```python
from build123d import *

# Parameters (mm, degrees)
F0_W     = 110
F0_H     = 120
F1_DEPTH = 2
F2_R     = 1.5
F3_W     = 2
F3_H     = 2
F3_R     = 1.75
F4_DEPTH = 2
F5_R     = 3


with BuildPart() as f1:
    # F0 (on Top) → F1 (new body)
    with BuildSketch(Plane.XY):
        Rectangle(F0_W, F0_H)
        with BuildLine():
            ThreePointArc((-50, 52.75), (-51.5909902577, 56.5909902577), (-47.75, 55))
            Line((-47.75, 55), (47.75, 55))
            ThreePointArc((47.75, 55), (50, 57.25), (52.25, 55))
            ThreePointArc((52.25, 55), (51.5909902577, 53.4090097423), (50, 52.75))
            Line((50, 52.75), (50, -42.75))
            ThreePointArc((50, -42.75), (51.5909902577, -43.4090097423), (52.25, -45))
            ThreePointArc((52.25, -45), (50, -47.25), (47.75, -45))
            Line((47.75, -45), (-47.75, -45))
            ThreePointArc((-47.75, -45), (-51.5909902577, -46.5909902577), (-50, -42.75))
            Line((-50, -42.75), (-50, 52.75))
        make_face(mode=Mode.SUBTRACT)
        with BuildLine():
            Line((47.75, 55), (-47.75, 55))
            ThreePointArc((-47.75, 55), (-48.4090097423, 53.4090097423), (-50, 52.75))
            Line((-50, 52.75), (-50, -42.75))
            ThreePointArc((-50, -42.75), (-48.4090097423, -43.4090097423), (-47.75, -45))
            Line((-47.75, -45), (47.75, -45))
            ThreePointArc((47.75, -45), (48.4090097423, -43.4090097423), (50, -42.75))
            Line((50, -42.75), (50, 52.75))
            ThreePointArc((50, 52.75), (48.4090097423, 53.4090097423), (47.75, 55))
        make_face()
    extrude(amount=F1_DEPTH)

    # F2
    f2_edges = [f1.edges().sort_by_distance(p)[0] for p in [
        (55, 60, 1),
        (55, -60, 1),
        (-55, -60, 1),
        (-55, 60, 1),
    ]]
    fillet(f2_edges, radius=F2_R)

    # F3 (on face) → F4 (cut)
    with BuildSketch(Plane.XY.offset(2)):
        with Locations((-24, 1)):
            Rectangle(F3_W, F3_H)
        with Locations((-26, 1)):
            Rectangle(F3_W, F3_H)
        with BuildLine():
            Line((-27, 2), (-25, 2))
            Line((-25, 2), (-23, 2))
            Line((-23, 2), (-23, 7.5))
            ThreePointArc((-23, 7.5), (-25, 9.5), (-27, 7.5))
            Line((-27, 7.5), (-27, 2))
        make_face()
        with Locations((-24, -1)):
            Rectangle(F3_W, F3_H)
        with Locations((-26, -1)):
            Rectangle(F3_W, F3_H)
        with BuildLine():
            Line((-27, 0), (-27, 2))
            Line((-27, 2), (-32.5, 2))
            ThreePointArc((-32.5, 2), (-34.5, 0), (-32.5, -2))
            Line((-32.5, -2), (-27, -2))
            Line((-27, -2), (-27, 0))
        make_face()
        with BuildLine():
            Line((-17.5, 2), (-23, 2))
            Line((-23, 2), (-23, 0))
            Line((-23, 0), (-23, -2))
            Line((-23, -2), (-17.5, -2))
            ThreePointArc((-17.5, -2), (-15.5, 0), (-17.5, 2))
        make_face()
        with BuildLine():
            Line((-23, -2), (-25, -2))
            Line((-25, -2), (-27, -2))
            Line((-27, -2), (-27, -7.5))
            ThreePointArc((-27, -7.5), (-25, -9.5), (-23, -7.5))
            Line((-23, -7.5), (-23, -2))
        make_face()
        Circle(F3_R)
        with BuildLine():
            Line((23, 2), (17.5, 2))
            ThreePointArc((17.5, 2), (15.5, 0), (17.5, -2))
            Line((17.5, -2), (23, -2))
            Line((23, -2), (23, 0))
            Line((23, 0), (23, 2))
        make_face()
        with BuildLine():
            Line((23, 7.5), (23, 2))
            Line((23, 2), (25, 2))
            Line((25, 2), (27, 2))
            Line((27, 2), (27, 7.5))
            ThreePointArc((27, 7.5), (25, 9.5), (23, 7.5))
        make_face()
        with Locations((24, 1)):
            Rectangle(F3_W, F3_H)
        with Locations((26, 1)):
            Rectangle(F3_W, F3_H)
        with Locations((24, -1)):
            Rectangle(F3_W, F3_H)
        with BuildLine():
            Line((25, -2), (23, -2))
            Line((23, -2), (23, -7.5))
            ThreePointArc((23, -7.5), (25, -9.5), (27, -7.5))
            Line((27, -7.5), (27, -2))
            Line((27, -2), (25, -2))
        make_face()
        with BuildLine():
            Line((32.5, 2), (27, 2))
            Line((27, 2), (27, 0))
            Line((27, 0), (27, -2))
            Line((27, -2), (32.5, -2))
            ThreePointArc((32.5, -2), (34.5, 0), (32.5, 2))
        make_face()
        with Locations((26, -1)):
            Rectangle(F3_W, F3_H)
        with Locations((1, 26)):
            Rectangle(F3_W, F3_H)
        with Locations((-1, 26)):
            Rectangle(F3_W, F3_H)
        with BuildLine():
            Line((-2, 27), (0, 27))
            Line((0, 27), (2, 27))
            Line((2, 27), (2, 32.5))
            ThreePointArc((2, 32.5), (0, 34.5), (-2, 32.5))
            Line((-2, 32.5), (-2, 27))
        make_face()
        with Locations((1, 24)):
            Rectangle(F3_W, F3_H)
        with Locations((-1, 24)):
            Rectangle(F3_W, F3_H)
        with BuildLine():
            Line((-2, 25), (-2, 27))
            Line((-2, 27), (-7.5, 27))
            ThreePointArc((-7.5, 27), (-9.5, 25), (-7.5, 23))
            Line((-7.5, 23), (-2, 23))
            Line((-2, 23), (-2, 25))
        make_face()
        with BuildLine():
            Line((7.5, 27), (2, 27))
            Line((2, 27), (2, 25))
            Line((2, 25), (2, 23))
            Line((2, 23), (7.5, 23))
            ThreePointArc((7.5, 23), (9.5, 25), (7.5, 27))
        make_face()
        with BuildLine():
            Line((2, 23), (0, 23))
            Line((0, 23), (-2, 23))
            Line((-2, 23), (-2, 17.5))
            ThreePointArc((-2, 17.5), (0, 15.5), (2, 17.5))
            Line((2, 17.5), (2, 23))
        make_face()
        with BuildLine():
            ThreePointArc((-2, -32.5), (0, -34.5), (2, -32.5))
            Line((2, -32.5), (2, -27))
            Line((2, -27), (0, -27))
            Line((0, -27), (-2, -27))
            Line((-2, -27), (-2, -32.5))
        make_face()
        with Locations((1, -26)):
            Rectangle(F3_W, F3_H)
        with BuildLine():
            Line((2, -25), (2, -27))
            Line((2, -27), (7.5, -27))
            ThreePointArc((7.5, -27), (9.5, -25), (7.5, -23))
            Line((7.5, -23), (2, -23))
            Line((2, -23), (2, -25))
        make_face()
        with Locations((-1, -26)):
            Rectangle(F3_W, F3_H)
        with BuildLine():
            Line((-7.5, -27), (-2, -27))
            Line((-2, -27), (-2, -25))
            Line((-2, -25), (-2, -23))
            Line((-2, -23), (-7.5, -23))
            ThreePointArc((-7.5, -23), (-9.5, -25), (-7.5, -27))
        make_face()
        with Locations((1, -24)):
            Rectangle(F3_W, F3_H)
        with Locations((-1, -24)):
            Rectangle(F3_W, F3_H)
        with BuildLine():
            Line((0, -23), (2, -23))
            Line((2, -23), (2, -17.5))
            ThreePointArc((2, -17.5), (0, -15.5), (-2, -17.5))
            Line((-2, -17.5), (-2, -23))
            Line((-2, -23), (0, -23))
        make_face()
    extrude(amount=-F4_DEPTH, mode=Mode.SUBTRACT)

    # F5
    f5_edges = [f1.edges().sort_by_distance(p)[0] for p in [
        (-23, -2, 1),
        (-23, 2, 1),
        (-27, -2, 1),
        (-27, 2, 1),
        (23, 2, 1),
        (23, -2, 1),
        (27, 2, 1),
        (27, -2, 1),
        (-2, 27, 1),
        (2, 27, 1),
        (2, 23, 1),
        (-2, 23, 1),
        (-2, -23, 1),
        (-2, -27, 1),
        (2, -27, 1),
        (2, -23, 1),
    ]]
    fillet(f5_edges, radius=F5_R)


solid = f1.part
```
Read the model definition and answer for the solid it produces. Units are mm, in the model's axes. A direction names the side the tool comes from. Give positions to 0.01 mm unless a question says otherwise; leave off trailing zeros. Order: outer loops, then holes, each group sorted by start corner. A loop starts at its lowest first (then second) coordinate and runs counter-clockwise, first axis right, second up.
(1) Given pin 1 (4 mm diameter, centred on x = 0, y = 0, fed in from -Z), flat-ended and moving along its own axis, determine where the tip first touches the part or whether it passes through.
(2) For faces 3 (the cylindrical face through (27.9, 2.86, 0.99)), 4 (the flat face through (-1, -12, 2)), determine the directions among +Z, -Z, +X, -X, +Y, -Y from which every point of the face is accessible in a straight line to the end or side of a thin tool.
(3) Straight lines are drawn through the part: L1, parallel to Y at x = -50, z = 1.15; L2, parallel to X at y = -6, z = 1.4; L3, parallel to Y at x = 0, z = 0.5. For each, find the intervals that lie inside material, in ascending order.
(4) For a pull along Y with two mould halves and no side action, classify faces 1 (the flat face through (-1, -12, 0)), 2 (the cylindrical face through (22.1, -2.86, 0.99)) as released by +Y, released by -Y, zero draft, split by the parting line, or undercut.
(5) Find section A-A (y = 25). Give the vertices of the cut face in (x, z).
(6) Find section B-B (z = 0.55). Give the number of separate pieces and of enclosed holes in the cut face, plus the area to 3 significant figures.
Result sheet:
1. pin 1: stops at z = 0
2. face 3: +Z, -Z
2. face 4: +Z, +X, -X, +Y, -Y
3. L1: y = -60 to -47.25, -42.75 to 52.75, 57.25 to 60
3. L2: x = -55 to -27, -23 to 23, 27 to 55
3. L3: y = -60 to -34.5, -15.5 to -1.75, 1.75 to 15.5, 34.5 to 60
4. face 1: zero draft
4. face 2: undercut
5. outline: (-55, 0) - (-9.5, 0) - (-9.5, 2) - (-55, 2) - close; (9.5, 0) - (55, 0) - (55, 2) - (9.5, 2) - close
6. separate pieces: 1
6. enclosed holes: 9
6. area: 12,600 mm2
